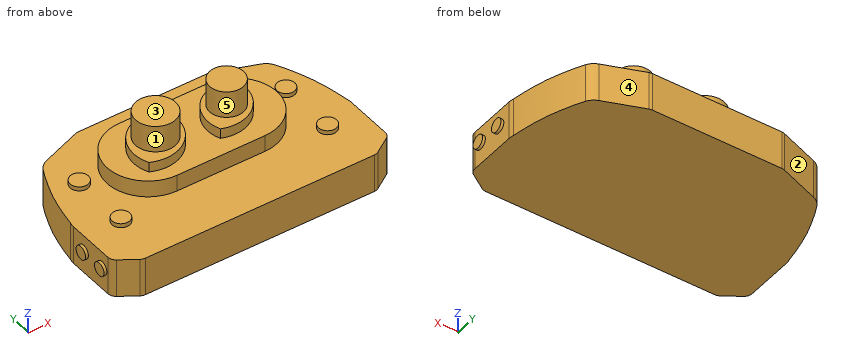
```python
from build123d import *

# Parameters (mm, degrees)
BOSS_EXTRUDE1_DEPTH = 23
SKETCH5_R           = 4
BOSS_EXTRUDE3_DEPTH = 1.7
SKETCH8_R           = 4
BOSS_EXTRUDE4_DEPTH = 1.7
SKETCH12_R          = 5.309585237
SKETCH12_R_2        = 5.383577716
SKETCH12_R_3        = 5.290961271
SKETCH12_R_4        = 5.444301549
BOSS_EXTRUDE5_DEPTH = 9.9
BOSS_EXTRUDE6_DEPTH = 22
CUT_EXTRUDE1_START  = -16
SKETCH16_R          = 11.94
CUT_EXTRUDE1_DEPTH  = 16
CUT_EXTRUDE2_START  = -16
SKETCH17_R          = 10.13
CUT_EXTRUDE2_DEPTH  = 16
CUT_EXTRUDE3_START  = -7.4
SKETCH18_R          = 5.309585237
CUT_EXTRUDE3_DEPTH  = 7.4
CUT_EXTRUDE4_START  = -7.4
SKETCH19_R          = 5.383577716
CUT_EXTRUDE4_DEPTH  = 7.4
CUT_EXTRUDE5_START  = -7.4
SKETCH20_R          = 5.444301549
CUT_EXTRUDE5_DEPTH  = 7.4
CUT_EXTRUDE6_START  = -7.4
SKETCH21_R          = 5.290961271
CUT_EXTRUDE6_DEPTH  = 7.4


with BuildPart() as part:
    # Sketch2 → Boss-Extrude1 (new body)
    with BuildSketch(Plane.XY):
        with BuildLine():
            Line((70.523413182, -121.258597495), (80.001788964, -115.008475165))
            ThreePointArc((80.001788964, -115.008475165), (81.651709385, -113.204688447), (82.249297777, -110.834293536))
            Line((82.249297777, -110.834293536), (82.249297777, -82.060728072))
            ThreePointArc((82.249297777, -82.060728072), (82.132627635, -80.537642087), (81.785339594, -79.050095835))
            add(Edge.make_bspline(
                [(81.785339594, -79.050095835), (81.779550585, -79.03175941), (79.763594577, -64.21980724), (72.310783114, -44.632084365), (70.089271073, -39.87053002), (68.584818962, -37.26596578)],
                knots=[0.01010668, 0.01010668, 0.01010668, 0.01010668, 0.430228508, 0.512694162, 0.834763224, 0.834763224, 0.834763224, 0.834763224], degree=3))
            ThreePointArc((68.584818962, -37.26596578), (66.377835563, -34.627803803), (63.407507036, -32.893496223))
            Line((63.407507036, -32.893496223), (39.759590264, -24.109812278))
            ThreePointArc((39.759590264, -24.109812278), (38.90305511, -23.875770322), (38.018627658, -23.796927511))
            Line((38.018627658, -23.796927511), (-39.520032104, -23.796927511))
            ThreePointArc((-39.520032104, -23.796927511), (-40.404459556, -23.875770322), (-41.26099471, -24.109812278))
            Line((-41.26099471, -24.109812278), (-64.908911482, -32.893496223))
            ThreePointArc((-64.908911482, -32.893496223), (-67.879240009, -34.627803803), (-70.086223408, -37.26596578))
            add(Edge.make_bspline(
                [(-83.28674404, -79.050095835), (-83.280955031, -79.03175941), (-81.264999023, -64.21980724), (-73.81218756, -44.632084365), (-71.590675519, -39.87053002), (-70.086223408, -37.26596578)],
                knots=[0.01010668, 0.01010668, 0.01010668, 0.01010668, 0.430228508, 0.512694162, 0.834763224, 0.834763224, 0.834763224, 0.834763224], degree=3))
            ThreePointArc((-83.28674404, -79.050095835), (-83.634032081, -80.537642087), (-83.750702223, -82.060728072))
            Line((-83.750702223, -82.060728072), (-83.750702223, -110.834293536))
            ThreePointArc((-83.750702223, -110.834293536), (-83.153113831, -113.204688447), (-81.50319341, -115.008475165))
            Line((-81.50319341, -115.008475165), (-72.024817629, -121.258597495))
            ThreePointArc((-72.024817629, -121.258597495), (-70.709179228, -121.873513284), (-69.272326442, -122.084415867))
            Line((-69.272326442, -122.084415867), (67.770921996, -122.084415867))
            ThreePointArc((67.770921996, -122.084415867), (69.207774782, -121.873513284), (70.523413182, -121.258597495))
        make_face()
    extrude(amount=BOSS_EXTRUDE1_DEPTH)

    # Sketch5 → Boss-Extrude3 (add)
    with BuildSketch(Plane.ZY.offset(83.750702223)):
        with Locations(Location((13.083649818, -90.551709518, 0), (0, 0, 90))):
            Circle(SKETCH5_R)
        with Locations(Location((13.083649818, -106.069633318, 0), (0, 0, 90))):
            Circle(SKETCH5_R)
    extrude(amount=BOSS_EXTRUDE3_DEPTH)

    # Sketch8 → Boss-Extrude4 (add)
    with BuildSketch(Plane(origin=(82.249297777, 0, 0), x_dir=(0, 0, -1), z_dir=(1, 0, 0))):
        with Locations(Location((-13.08, -90.550728072, 0), (0, 0, 270))):
            Circle(SKETCH8_R)
        with Locations(Location((-13.08, -106.070728072, 0), (0, 0, 270))):
            Circle(SKETCH8_R)
    extrude(amount=BOSS_EXTRUDE4_DEPTH)

    # Sketch12 → Boss-Extrude5 (add)
    with BuildSketch(Plane.XY.offset(23)):
        with Locations(Location((61.412858859, -56.74856372, 0), (0, 0, 180))):
            Circle(SKETCH12_R)
        with Locations(Location((61.412858859, -91.784557501, 0), (0, 0, 180))):
            Circle(SKETCH12_R_2)
        with Locations(Location((-62.293922582, -91.784557501, 0), (0, 0, 180))):
            Circle(SKETCH12_R_3)
        with Locations(Location((-62.293922582, -56.74856372, 0), (0, 0, 180))):
            Circle(SKETCH12_R_4)
        with BuildLine():
            Line((26.03317791, -39.941081705), (-26.605656617, -39.941081705))
            ThreePointArc((-26.605656617, -39.941081705), (-51.069934746, -64.405359834), (-26.605656617, -88.869637962))
            Line((-26.605656617, -88.869637962), (26.03317791, -88.869637962))
            ThreePointArc((26.03317791, -88.869637962), (50.497456038, -64.405359834), (26.03317791, -39.941081705))
        make_face()
    extrude(amount=BOSS_EXTRUDE5_DEPTH)

    # Sketch15 → Boss-Extrude6 (add)
    with BuildSketch(Plane.XY.offset(32.9)):
        with BuildLine():
            ThreePointArc((-36.30694092, -78.897586955), (-32.416918561, -54.237740907), (-7.831564022, -49.901772358))
            ThreePointArc((-7.831564022, -49.901772358), (-11.721586381, -74.561618406), (-36.30694092, -78.897586955))
        make_face()
        with BuildLine():
            ThreePointArc((33.947027157, -50.665986501), (29.727203797, -73.404384895), (7.056950152, -77.976175614))
            ThreePointArc((7.056950152, -77.976175614), (11.276773512, -55.23777722), (33.947027157, -50.665986501))
        make_face()
    extrude(amount=BOSS_EXTRUDE6_DEPTH)

    # Sketch16 → Cut-Extrude1 (cut)
    with BuildSketch(Plane.XY.offset(54.9).offset(CUT_EXTRUDE1_START)):
        with BuildLine():
            ThreePointArc((-36.30694092, -78.897586955), (-32.416918561, -54.237740907), (-7.831564022, -49.901772358))
            ThreePointArc((-7.831564022, -49.901772358), (-11.721586381, -74.561618406), (-36.30694092, -78.897586955))
        make_face()
        with Locations((-22.069252471, -64.399679657)):
            Circle(SKETCH16_R, mode=Mode.SUBTRACT)
    extrude(amount=CUT_EXTRUDE1_DEPTH, mode=Mode.SUBTRACT)

    # Sketch17 → Cut-Extrude2 (cut)
    with BuildSketch(Plane.XY.offset(54.9).offset(CUT_EXTRUDE2_START)):
        with BuildLine():
            ThreePointArc((7.056950152, -77.976175614), (11.276773512, -55.23777722), (33.947027157, -50.665986501))
            ThreePointArc((33.947027157, -50.665986501), (29.727203797, -73.404384895), (7.056950152, -77.976175614))
        make_face()
        with Locations((20.501988655, -64.321081058)):
            Circle(SKETCH17_R, mode=Mode.SUBTRACT)
    extrude(amount=CUT_EXTRUDE2_DEPTH, mode=Mode.SUBTRACT)

    # Sketch18 → Cut-Extrude3 (cut)
    with BuildSketch(Plane.XY.offset(32.9).offset(CUT_EXTRUDE3_START)):
        with Locations(Location((61.412858859, -56.74856372, 0), (0, 0, 180))):
            Circle(SKETCH18_R)
    extrude(amount=CUT_EXTRUDE3_DEPTH, mode=Mode.SUBTRACT)

    # Sketch19 → Cut-Extrude4 (cut)
    with BuildSketch(Plane.XY.offset(32.9).offset(CUT_EXTRUDE4_START)):
        with Locations(Location((61.412858859, -91.784557501, 0), (0, 0, 180))):
            Circle(SKETCH19_R)
    extrude(amount=CUT_EXTRUDE4_DEPTH, mode=Mode.SUBTRACT)

    # Sketch20 → Cut-Extrude5 (cut)
    with BuildSketch(Plane.XY.offset(32.9).offset(CUT_EXTRUDE5_START)):
        with Locations(Location((-62.293922582, -56.74856372, 0), (0, 0, 180))):
            Circle(SKETCH20_R)
    extrude(amount=CUT_EXTRUDE5_DEPTH, mode=Mode.SUBTRACT)

    # Sketch21 → Cut-Extrude6 (cut)
    with BuildSketch(Plane.XY.offset(32.9).offset(CUT_EXTRUDE6_START)):
        with Locations(Location((-62.293922582, -91.784557501, 0), (0, 0, 180))):
            Circle(SKETCH21_R)
    extrude(amount=CUT_EXTRUDE6_DEPTH, mode=Mode.SUBTRACT)


solid = part.part
```
For this review, take the finished solid that the model builds, in its own axes (mm). Face numbers are marked on the shaded views. A direction names the side the tool comes from. Give positions to 0.01 mm unless a question says otherwise; leave off trailing zeros. Order: outer loops, then holes, each group sorted by start corner. A loop starts at its lowest first (then second) coordinate and runs counter-clockwise, first axis right, second up.
1) Insertion check: pin 1 (12 mm diameter, centred on y = -60.5, z = 29.5, fed in from -X); pin 2 (6 mm diameter, centred on x = 22, y = -37, fed in from +Z); pin 3 (3.5 mm diameter, centred on x = -61, y = -56.5, fed in from +Z). Each pin has a flat end and moves straight along its axis. Give the tip position at first contact, or say it passes through.
2) Take a section at D-D (z = 50.5). Give the boundary of the cut face in (x, y).
3) Wall thickness on line 1 (Z direction, x = -29, y = -52); line 2 (Z direction, x = -34, y = -108); line 3 (X direction, y = -56, z = 43): over which ranges is each line inside the solid? List them lowest first.
4) Take a section at B-B (x = -62). Give the boundary of the cut face in (y, z).
5) The part is to be moulded in two halves that separate along X. For the marked faces 3, 4 and 5, say which applies: released by +X, released by -X, zero draft, split by the parting line, or undercut.
6) For the marked faces 1 and 2, list the 3-axis set-ups (+Z, -Z, +X, -X, +Y, -Y) from which the entire face can be reached by the end or side of a thin tool; tool diameter is ignored.
7) Take a section at C-C (z = 31). Give the boundary of the cut face in (x, y), then the cut area to 3 significant figures.
8) Take a section at A-A (y = -106). Give the boundary of the cut face in (x, z), then the cut area to 3 significant figures.
Derived:
1. pin 1: stops at x = -67.74
1. pin 2: stops at z = 32.9
1. pin 3: stops at z = 25.5
2. outline: circle Ø23.88 at (-22.07, -64.4); circle Ø20.26 at (20.5, -64.32)
3. line 1: z = 0 to 38.9
3. line 2: z = 0 to 23
3. line 3: x = -30.56 to -13.58, 14.72 to 26.28
4. outline: (-122.08, 0) - (-31.81, 0) - (-31.81, 23) - (-51.31, 23) - (-51.31, 25.5) - (-62.18, 25.5) - (-62.18, 23) - (-86.5, 23) - (-86.5, 25.5) - (-97.07, 25.5) - (-97.07, 23) - (-122.08, 23) - close
5. face 3: zero draft
5. face 4: released by +X
5. face 5: undercut
6. face 1: +Z
6. face 2: +Z, -Z, -X, +Y
7. outline: (-26.61, -88.87) - (26.03, -88.87) arc R24.46 ccw to (26.03, -39.94) - (-26.61, -39.94) arc R24.46 ccw to start
7. area: 4,460 mm2
8. outline: (-85.45, 9.08) - (-83.75, 9.08) - (-83.75, 0) - (82.25, 0) - (82.25, 9.08) - (83.95, 9.08) - (83.95, 17.08) - (82.25, 17.08) - (82.25, 23) - (-83.75, 23) - (-83.75, 17.08) - (-85.45, 17.08) - close
8. area: 3,850 mm2
